from build123d import *

# Parameters (mm, degrees)
SKETCH_1_R      = 11
SKETCH_1_R_2    = 8.4
EXTRUDE_1_DEPTH = 2
SKETCH_2_R      = 9.6
SKETCH_2_R_2    = 7
EXTRUDE_2_DEPTH = 30
CHAMFER_1_SIZE  = 0.5
SKETCH_3_R      = 11
SKETCH_3_R_2    = 9.6
EXTRUDE_3_DEPTH = 10.8
CHAMFER_2_SIZE  = 1
CHAMFER_3_SIZE  = 0.3
CHAMFER_4_SIZE  = 0.5


with BuildPart() as part:
    # 스케치1 → 보스-돌출1 (new body)
    with BuildSketch(Plane.XY):
        Circle(SKETCH_1_R)
        Circle(SKETCH_1_R_2, mode=Mode.SUBTRACT)
    extrude(amount=EXTRUDE_1_DEPTH)

    # 스케치2 → 보스-돌출2 (add)
    with BuildSketch(Plane.XY.offset(2)):
        Circle(SKETCH_2_R)
        Circle(SKETCH_2_R_2, mode=Mode.SUBTRACT)
    extrude(amount=EXTRUDE_2_DEPTH)

    # 모따기1
    chamfer_1_edges = [part.edges().sort_by_distance(p)[0] for p in [
        (-8.4, 0, 0),
    ]]
    chamfer(chamfer_1_edges, length=CHAMFER_1_SIZE)

    # 스케치3 → 보스-돌출3 (add)
    with BuildSketch(Plane.XY.offset(2)):
        Circle(SKETCH_3_R)
        Circle(SKETCH_3_R_2, mode=Mode.SUBTRACT)
    extrude(amount=EXTRUDE_3_DEPTH)

    # 모따기2
    chamfer_2_edges = [part.edges().sort_by_distance(p)[0] for p in [
        (-9.6, 0, 32),
    ]]
    chamfer(chamfer_2_edges, length=CHAMFER_2_SIZE)

    # 모따기3
    chamfer_3_edges = [part.edges().sort_by_distance(p)[0] for p in [
        (-8.4, 0, 2),
    ]]
    chamfer(chamfer_3_edges, length=CHAMFER_3_SIZE)

    # 모따기4
    chamfer_4_edges = [part.edges().sort_by_distance(p)[0] for p in [
        (-11, 0, 0),
    ]]
    chamfer(chamfer_4_edges, length=CHAMFER_4_SIZE)


solid = part.part
Geometry: final body of the model. Coordinates: model frame, mm. A direction names the side the tool comes from. Coordinates: 2 decimals unless noted, no trailing zeros. Order: outer loops, then holes, each group sorted by start corner. A loop starts at its lowest first (then second) coordinate and runs counter-clockwise, first axis right, second up. Notation, with made-up numbers: M 15.5,81 L 37.5,81 A11 cw 37.5,101 Z; hole C 61,5 d11. An arc over 180 degrees is marked long. One line per question, with ' | ' between items. Start each with the question number.
Item 1: Cut plane C-C, the plane z = 25.5. Return the cut outline in (x, y), then the cut area to 3 significant figures.
Item 2: Cut plane A-A, the plane x = 0. Return the cut outline in (y, z).
Item 3: Cut plane D-D, the plane z = 12. Return the cut outline in (x, y).
Item 4: Set-up query: faces 1 (the cylindrical face through (8.012, 2.523, 1.092)), 2 (the flat face through (2, -7, 32)). Return all of +Z, -Z, +X, -X, +Y, -Y with unobstructed straight access to the full face (end or side cutting, diameter ignored); none if empty.
Item 5: Draft query along Y for faces 3 (the cylindrical face through (5.161, 8.095, 21.773)), 4 (the flat face through (1, 10, 12.8)), 5 (the cylindrical face through (6.466, -2.681, 16.79)). Return one class per face: released by +Y, released by -Y, zero draft, split by the parting line, or undercut.
Item 6: Ray query, probe 1 along Y at (x, z) = (0, 16.25); probe 2 along Y at (x, z) = (0, 10.25); probe 3 along Z at (x, y) = (7.75, -1). Return the intervals inside material, ascending. Write a range as [from, to].
Item 7: Pin query (flat end, axial travel): pin 1 Ø4 at (x, y) = (-1, -4) entering from -Z; pin 2 Ø1 at (x, z) = (-4, 16.5) entering from -Y; pin 3 Ø6 at (x, z) = (-5.5, 11) entering from -Y; pin 4 Ø3 at (x, z) = (-0.5, 28.5) entering from +Y. Return the tip coordinate at first contact, or that it passes through.
A:
1) outline: C 0,0 d19.2; hole C 0,0 d14 | area: 136 mm2
2) outline: M -11,0.5 L -10.5,0 L -8.9,0 L -8.4,0.5 L -8.4,1.7 L -8.1,2 L -7,2 L -7,32 L -8.6,32 L -9.6,31 L -9.6,12.8 L -11,12.8 Z; M 7,2 L 8.1,2 L 8.4,1.7 L 8.4,0.5 L 8.9,0 L 10.5,0 L 11,0.5 L 11,12.8 L 9.6,12.8 L 9.6,31 L 8.6,32 L 7,32 Z
3) outline: C 0,0 d22; hole C 0,0 d14
4) face 1: -Z | face 2: +Z, +X, -X, +Y, -Y
5) face 3: split by the parting line | face 4: zero draft | face 5: undercut
6) probe 1: y = [-9.6, -7], [7, 9.6] | probe 2: y = [-11, -7], [7, 11] | probe 3: z = [2, 32]
7) pin 1: passes through | pin 2: stops at y = -8.94 | pin 3: stops at y = -10.71 | pin 4: stops at y = 9.6
